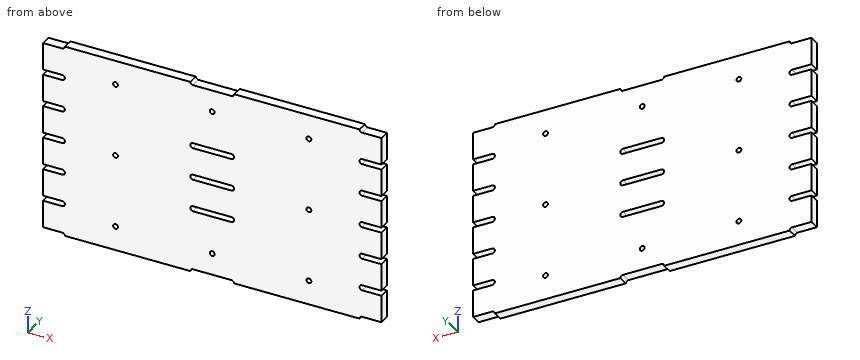
```python
from build123d import *

# Parameters (mm, degrees)
SKETCH1_W                  = 210
SKETCH1_H                  = 120
BOSS_EXTRUDE1_DEPTH        = 6.35
CUT_EXTRUDE1_DEPTH         = 122.100464491
LPATTERN1_COUNT            = 4
LPATTERN1_PITCH            = 20
LPATTERN1_COL_COUNT        = 4
LPATTERN1_COL_PITCH        = 20
LPATTERN2_COUNT            = 2
LPATTERN2_PITCH            = 105
LPATTERN2_COPY_1_DEPTH     = 122.100464491
LPATTERN2_COPY_2_DEPTH     = 122.100464491
LPATTERN2_COPY_3_DEPTH     = 122.100464491
LPATTERN2_COPY_4_DEPTH     = 122.100464491
LPATTERN2_COPY_5_DEPTH     = 122.100464491
LPATTERN2_COPY_6_DEPTH     = 122.100464491
LPATTERN2_COL_COUNT        = 2
LPATTERN2_COL_PITCH        = 105
LPATTERN2_COL_COPY_1_DEPTH = 122.100464491
LPATTERN2_COL_COPY_2_DEPTH = 122.100464491
LPATTERN2_COL_COPY_3_DEPTH = 122.100464491
LPATTERN2_COL_COPY_4_DEPTH = 122.100464491
LPATTERN2_COL_COPY_5_DEPTH = 122.100464491
LPATTERN2_COL_COPY_6_DEPTH = 122.100464491
SKETCH6_R                  = 1.5
CUT_EXTRUDE3_DEPTH         = 10
SKETCH7_R                  = 1.5
CUT_EXTRUDE4_DEPTH         = 10
BOSS_EXTRUDE2_DEPTH        = 6.35


with BuildPart() as part:
    # Sketch1 → Boss-Extrude1 (new body)
    with BuildSketch(Plane(origin=(0, 0, 0), x_dir=(1, 0, 0), z_dir=(0, 1, 0))):
        Rectangle(SKETCH1_W, SKETCH1_H)
    extrude(amount=BOSS_EXTRUDE1_DEPTH)

    # Sketch3 → Cut-Extrude1 (cut, symmetric)
    with BuildSketch(Plane(origin=(0, 6.35, 0), x_dir=(1, 0, 0), z_dir=(0, 1, 0))):
        with BuildLine():
            Line((12, -1.6), (-12, -1.6))
            ThreePointArc((-12, -1.6), (-13.6, 0), (-12, 1.6))
            Line((-12, 1.6), (12, 1.6))
            ThreePointArc((12, 1.6), (13.6, 0), (12, -1.6))
        make_face()
    cut_extrude1 = extrude(amount=CUT_EXTRUDE1_DEPTH, both=True, mode=Mode.SUBTRACT)

    # LPattern1: Cut-Extrude1 ×4
    with Locations(*[(0, 0, i * LPATTERN1_PITCH) for i in range(1, LPATTERN1_COUNT)]):
        add(cut_extrude1, mode=Mode.SUBTRACT)

    # LPattern1 col: Cut-Extrude1 ×4
    with Locations(*[(0, 0, -i * LPATTERN1_COL_PITCH) for i in range(1, LPATTERN1_COL_COUNT)]):
        add(cut_extrude1, mode=Mode.SUBTRACT)

    # LPattern2: Cut-Extrude1 ×2
    with Locations(*[(i * LPATTERN2_PITCH, 0, 0) for i in range(1, LPATTERN2_COUNT)]):
        add(cut_extrude1, mode=Mode.SUBTRACT)

    # LPattern2 copy 1 sketch → LPattern2 copy 1 (cut, symmetric)
    with BuildSketch(Plane(origin=(105, 6.35, 20), x_dir=(1, 0, 0), z_dir=(0, 1, 0))):
        with BuildLine():
            Line((12, -1.6), (-12, -1.6))
            ThreePointArc((-12, -1.6), (-13.6, 0), (-12, 1.6))
            Line((-12, 1.6), (12, 1.6))
            ThreePointArc((12, 1.6), (13.6, 0), (12, -1.6))
        make_face()
    extrude(amount=LPATTERN2_COPY_1_DEPTH, both=True, mode=Mode.SUBTRACT)

    # LPattern2 copy 2 sketch → LPattern2 copy 2 (cut, symmetric)
    with BuildSketch(Plane(origin=(105, 6.35, 40), x_dir=(1, 0, 0), z_dir=(0, 1, 0))):
        with BuildLine():
            Line((12, -1.6), (-12, -1.6))
            ThreePointArc((-12, -1.6), (-13.6, 0), (-12, 1.6))
            Line((-12, 1.6), (12, 1.6))
            ThreePointArc((12, 1.6), (13.6, 0), (12, -1.6))
        make_face()
    extrude(amount=LPATTERN2_COPY_2_DEPTH, both=True, mode=Mode.SUBTRACT)

    # LPattern2 copy 3 sketch → LPattern2 copy 3 (cut, symmetric)
    with BuildSketch(Plane(origin=(105, 6.35, 60), x_dir=(1, 0, 0), z_dir=(0, 1, 0))):
        with BuildLine():
            Line((12, -1.6), (-12, -1.6))
            ThreePointArc((-12, -1.6), (-13.6, 0), (-12, 1.6))
            Line((-12, 1.6), (12, 1.6))
            ThreePointArc((12, 1.6), (13.6, 0), (12, -1.6))
        make_face()
    extrude(amount=LPATTERN2_COPY_3_DEPTH, both=True, mode=Mode.SUBTRACT)

    # LPattern2 copy 4 sketch → LPattern2 copy 4 (cut, symmetric)
    with BuildSketch(Plane(origin=(105, 6.35, -20), x_dir=(1, 0, 0), z_dir=(0, 1, 0))):
        with BuildLine():
            Line((12, -1.6), (-12, -1.6))
            ThreePointArc((-12, -1.6), (-13.6, 0), (-12, 1.6))
            Line((-12, 1.6), (12, 1.6))
            ThreePointArc((12, 1.6), (13.6, 0), (12, -1.6))
        make_face()
    extrude(amount=LPATTERN2_COPY_4_DEPTH, both=True, mode=Mode.SUBTRACT)

    # LPattern2 copy 5 sketch → LPattern2 copy 5 (cut, symmetric)
    with BuildSketch(Plane(origin=(105, 6.35, -40), x_dir=(1, 0, 0), z_dir=(0, 1, 0))):
        with BuildLine():
            Line((12, -1.6), (-12, -1.6))
            ThreePointArc((-12, -1.6), (-13.6, 0), (-12, 1.6))
            Line((-12, 1.6), (12, 1.6))
            ThreePointArc((12, 1.6), (13.6, 0), (12, -1.6))
        make_face()
    extrude(amount=LPATTERN2_COPY_5_DEPTH, both=True, mode=Mode.SUBTRACT)

    # LPattern2 copy 6 sketch → LPattern2 copy 6 (cut, symmetric)
    with BuildSketch(Plane(origin=(105, 6.35, -60), x_dir=(1, 0, 0), z_dir=(0, 1, 0))):
        with BuildLine():
            Line((12, -1.6), (-12, -1.6))
            ThreePointArc((-12, -1.6), (-13.6, 0), (-12, 1.6))
            Line((-12, 1.6), (12, 1.6))
            ThreePointArc((12, 1.6), (13.6, 0), (12, -1.6))
        make_face()
    extrude(amount=LPATTERN2_COPY_6_DEPTH, both=True, mode=Mode.SUBTRACT)

    # LPattern2 col: Cut-Extrude1 ×2
    with Locations(*[(-i * LPATTERN2_COL_PITCH, 0, 0) for i in range(1, LPATTERN2_COL_COUNT)]):
        add(cut_extrude1, mode=Mode.SUBTRACT)

    # LPattern2 col copy 1 sketch → LPattern2 col copy 1 (cut, symmetric)
    with BuildSketch(Plane(origin=(-105, 6.35, 20), x_dir=(1, 0, 0), z_dir=(0, 1, 0))):
        with BuildLine():
            Line((12, -1.6), (-12, -1.6))
            ThreePointArc((-12, -1.6), (-13.6, 0), (-12, 1.6))
            Line((-12, 1.6), (12, 1.6))
            ThreePointArc((12, 1.6), (13.6, 0), (12, -1.6))
        make_face()
    extrude(amount=LPATTERN2_COL_COPY_1_DEPTH, both=True, mode=Mode.SUBTRACT)

    # LPattern2 col copy 2 sketch → LPattern2 col copy 2 (cut, symmetric)
    with BuildSketch(Plane(origin=(-105, 6.35, 40), x_dir=(1, 0, 0), z_dir=(0, 1, 0))):
        with BuildLine():
            Line((12, -1.6), (-12, -1.6))
            ThreePointArc((-12, -1.6), (-13.6, 0), (-12, 1.6))
            Line((-12, 1.6), (12, 1.6))
            ThreePointArc((12, 1.6), (13.6, 0), (12, -1.6))
        make_face()
    extrude(amount=LPATTERN2_COL_COPY_2_DEPTH, both=True, mode=Mode.SUBTRACT)

    # LPattern2 col copy 3 sketch → LPattern2 col copy 3 (cut, symmetric)
    with BuildSketch(Plane(origin=(-105, 6.35, 60), x_dir=(1, 0, 0), z_dir=(0, 1, 0))):
        with BuildLine():
            Line((12, -1.6), (-12, -1.6))
            ThreePointArc((-12, -1.6), (-13.6, 0), (-12, 1.6))
            Line((-12, 1.6), (12, 1.6))
            ThreePointArc((12, 1.6), (13.6, 0), (12, -1.6))
        make_face()
    extrude(amount=LPATTERN2_COL_COPY_3_DEPTH, both=True, mode=Mode.SUBTRACT)

    # LPattern2 col copy 4 sketch → LPattern2 col copy 4 (cut, symmetric)
    with BuildSketch(Plane(origin=(-105, 6.35, -20), x_dir=(1, 0, 0), z_dir=(0, 1, 0))):
        with BuildLine():
            Line((12, -1.6), (-12, -1.6))
            ThreePointArc((-12, -1.6), (-13.6, 0), (-12, 1.6))
            Line((-12, 1.6), (12, 1.6))
            ThreePointArc((12, 1.6), (13.6, 0), (12, -1.6))
        make_face()
    extrude(amount=LPATTERN2_COL_COPY_4_DEPTH, both=True, mode=Mode.SUBTRACT)

    # LPattern2 col copy 5 sketch → LPattern2 col copy 5 (cut, symmetric)
    with BuildSketch(Plane(origin=(-105, 6.35, -40), x_dir=(1, 0, 0), z_dir=(0, 1, 0))):
        with BuildLine():
            Line((12, -1.6), (-12, -1.6))
            ThreePointArc((-12, -1.6), (-13.6, 0), (-12, 1.6))
            Line((-12, 1.6), (12, 1.6))
            ThreePointArc((12, 1.6), (13.6, 0), (12, -1.6))
        make_face()
    extrude(amount=LPATTERN2_COL_COPY_5_DEPTH, both=True, mode=Mode.SUBTRACT)

    # LPattern2 col copy 6 sketch → LPattern2 col copy 6 (cut, symmetric)
    with BuildSketch(Plane(origin=(-105, 6.35, -60), x_dir=(1, 0, 0), z_dir=(0, 1, 0))):
        with BuildLine():
            Line((12, -1.6), (-12, -1.6))
            ThreePointArc((-12, -1.6), (-13.6, 0), (-12, 1.6))
            Line((-12, 1.6), (12, 1.6))
            ThreePointArc((12, 1.6), (13.6, 0), (12, -1.6))
        make_face()
    extrude(amount=LPATTERN2_COL_COPY_6_DEPTH, both=True, mode=Mode.SUBTRACT)

    # Sketch6 → Cut-Extrude3 (cut)
    with BuildSketch(Plane(origin=(0, 6.35, 0), x_dir=(1, 0, 0), z_dir=(0, 1, 0))):
        with Locations(Location((-60, 45, 0), (0, 0, 270))):
            Circle(SKETCH6_R)
        with Locations(Location((60, 45, 0), (0, 0, 270))):
            Circle(SKETCH6_R)
        with Locations(Location((60, -45, 0), (0, 0, 270))):
            Circle(SKETCH6_R)
        with Locations(Location((-60, -45, 0), (0, 0, 270))):
            Circle(SKETCH6_R)
        with Locations(Location((0, 45, 0), (0, 0, 270))):
            Circle(SKETCH6_R)
        with Locations(Location((0, -45, 0), (0, 0, 270))):
            Circle(SKETCH6_R)
    extrude(amount=-CUT_EXTRUDE3_DEPTH, mode=Mode.SUBTRACT)

    # Sketch7 → Cut-Extrude4 (cut)
    with BuildSketch(Plane(origin=(0, 6.35, 0), x_dir=(1, 0, 0), z_dir=(0, 1, 0))):
        with Locations(Location((-60, 0, 0), (0, 0, 270))):
            Circle(SKETCH7_R)
        with Locations(Location((60, 0, 0), (0, 0, 270))):
            Circle(SKETCH7_R)
    extrude(amount=-CUT_EXTRUDE4_DEPTH, mode=Mode.SUBTRACT)

    # Sketch8 → Boss-Extrude2 (add)
    with BuildSketch(Plane(origin=(0, 6.35, 0), x_dir=(1, 0, 0), z_dir=(0, 1, 0))):
        with BuildLine():
            Line((-12, 42), (12, 42))
            ThreePointArc((12, 42), (14, 40), (12, 38))
            Line((12, 38), (-12, 38))
            ThreePointArc((-12, 38), (-14, 40), (-12, 42))
        make_face()
        with BuildLine():
            Line((-12, -38), (12, -38))
            ThreePointArc((12, -38), (14, -40), (12, -42))
            Line((12, -42), (-12, -42))
            ThreePointArc((-12, -42), (-14, -40), (-12, -38))
        make_face()
    extrude(amount=-BOSS_EXTRUDE2_DEPTH)


solid = part.part
```
Verification items for the finished model (mm, model axes). Round coordinates to 2 decimals unless told otherwise and drop trailing zeros. Answer as a JSON object with one key per item and string values. Group by question number.
Q1. Section check A-A, the plane y = 5.25. Give the number of separate pieces and of enclosed holes in the cut face, plus the area to 3 significant figures.
Q2. Thickness scan on line 1 (X direction, y = 3.5, z = -45); line 2 (Z direction, x = -7, y = 2.5); line 3 (X direction, y = 4.5, z = 0). Record the ranges inside material, lowest first.
Q3. Go/stop test with flat-tipped pins: pin 1 Ø1.9 at (x, y) = (-100, 2.5) entering from +Z; pin 2 Ø1.9 at (x, y) = (96, 2) entering from -Z. Record where each tip stops, or that it passes through.
Found:
{
 "1": {"separate pieces": "1", "enclosed holes": "11", "area": "24,300 mm^2"},
 "2": {"line 1": "x = -105 to -61.5, -58.5 to -1.5, 1.5 to 58.5, 61.5 to 105", "line 2": "z = -58.4 to -21.6, -18.4 to -1.6, 1.6 to 18.4, 21.6 to 58.4", "line 3": "x = -91.4 to -61.5, -58.5 to -13.6, 13.6 to 58.5, 61.5 to 91.4"},
 "3": {"pin 1": "stops at z = 58.4", "pin 2": "stops at z = -58.4"}
}
